Autodesk Inventor part; units mm, degrees
ref_plane "YZ Plane" through (0, 0, 0) normal (1, 0, 0) x (0, 1, 0)
ref_plane "XZ Plane" through (0, 0, 0) normal (0, 1, 0) x (-1, 0, 0)
ref_plane "XY Plane" through (0, 0, 0) normal (0, 0, 1) x (1, 0, 0)
ref_plane "Work Plane1" through (-11.5353, 732.2171, -211.5196) normal (-0.0000012, -0.9978756, -0.0651475) x (1, -0.0000012, -0.0000001)
sketch "Sketch2" plane through (-11.5353, 732.2171, -211.5196) normal (-0.0000012, -0.9978756, -0.0651475) x (1, -0.0000012, -0.0000001)
  line L0 (47.2205, 275.3712) -> (-77.9795, 275.3712)
  line L1 (-77.9795, 275.3712) -> (-77.9795, 150.1712)
  line L2 (-77.9795, 150.1712) -> (47.2205, 150.1712)
  line L3 (47.2205, 150.1712) -> (47.2205, 275.3712) construction
  line L4 (47.2205, 275.3712) -> (97.2205, 275.3712)
  line L5 (97.2205, 275.3712) -> (97.2205, 150.1712)
  line L6 (97.2205, 150.1712) -> (47.2205, 150.1712)
  line L7 (34.9205, 141.5153) -> (34.9205, 309.2543) construction
  line L8 (-65.6795, 309.2543) -> (-65.6795, 110.7061) construction
  line L9 (72.2205, 263.0712) -> (-113.8811, 263.0712) construction
  line L10 (72.2205, 162.4712) -> (-118.8511, 162.4712) construction
  point P0 (11.5362, 258.7723)
  point P1 (-138.0714, 537.573)
  point P2 (-211.9698, 678.1667)
  point P3 (34.9205, 263.0712)
  point P4 (34.9205, 162.4712)
  point P5 (-65.6795, 162.4712)
  point P6 (-65.6795, 263.0712)
  dimension "d15" = 125.2
  dimension "d16" = 125.2
  dimension "d23" = 50
  dimension "d30" = 12.3
  dimension "d31" = 100.6
  dimension "d32" = 12.3
  dimension "d33" = 100.6
extrude "Extrusion2" add sketch "Sketch2" along normal blind 6
hole "Hole1" at (23.3852, 715.0787, 50.9927) at (23.3852, 721.6325, -49.3936) at (-77.2148, 715.0788, 50.9927) direction (-0.0000012, -0.9978756, -0.0651475) diameter 5.1 end through all counterbore diameter 9.2 counterbore depth 2
hole "Hole2" at (-77.2148, 721.6326, -49.3935) direction (-0.0000012, -0.9978756, -0.0651475) diameter 7.2 end through all counterbore diameter 12.25 counterbore depth 2
properties part number "X axis carriage"
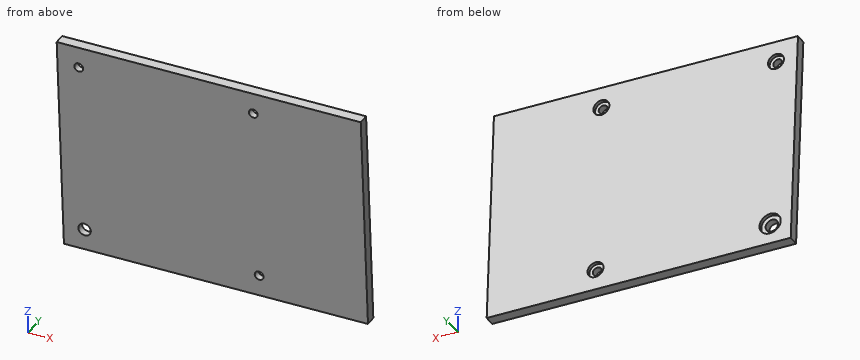
The model under review builds one solid part; all positions refer to its coordinate system, in mm. Round coordinates to 2 decimals unless told otherwise and drop trailing zeros. Write each loop counter-clockwise with the first axis right and the second up, starting at its lowest first coordinate (ties: lowest second). Pieces come first, ordered by that corner, then holes. Notation, with made-up numbers: M 20,34 L 40,34 A20 cw 40,57 Z; hole C 79,48 d7. An arc over 180 degrees is marked long. Answer as CSV lines item,"result". Start each with the question number.
Q1. Clearance check with flat-ended pins moving along their axes: P1, Ø5, axis at x = 26.5, z = 44.5, coming from the +Y side; P2, Ø1, axis at x = -5, z = 27, coming from the +Y side; P3, Ø12, axis at x = -39, z = -31.5, coming from the -Y side. State where each tip first meets the part, or that it passes through.
Q2. Wall thickness on line 1 along Y through (x, z) = (75, -47); line 2 along Y through (x, z) = (57.5, 18): over which ranges is each line inside the solid? List them lowest first.
Q3. Consider section B-B, the plane x = -68.5. Give the boundary of the cut face in (y, z).
Q4. Consider section A-A, the plane z = 5. Give the boundary of the cut face in (x, y), then the cut area to 3 significant figures.
Result set:
1,P1,"stops at y = 715.67"
1,P2,"stops at y = 716.68"
1,P3,"stops at y = 714.06"
2,line 1,"y = 715.46 to 721.48"
2,line 2,"y = 711.22 to 717.23"
3,outline,"M 708.29,62.88 L 716.45,-62.06 L 722.43,-61.67 L 714.28,63.27 Z"
4,outline,"M -89.51,712.07 L 85.69,712.07 L 85.69,718.08 L -89.51,718.08 Z"
4,area,"1,050 mm²"
